from build123d import *

# Parameters (mm, degrees)
CROQUIS1_R              = 27.5
CROQUIS1_R_2            = 19.05
SALIENTE_EXTRUIR1_DEPTH = 3
CORTAR_EXTRUIR1_DEPTH   = 3


with BuildPart() as part:
    # Croquis1 → Saliente-Extruir1 (new body)
    with BuildSketch(Plane(origin=(0, 0, 0), x_dir=(1, 0, 0), z_dir=(0, 1, 0))):
        Circle(CROQUIS1_R)
        Circle(CROQUIS1_R_2, mode=Mode.SUBTRACT)
    extrude(amount=SALIENTE_EXTRUIR1_DEPTH)

    # Croquis2 → Cortar-Extruir1 (cut)
    with BuildSketch(Plane(origin=(0, 3, 0), x_dir=(1, 0, 0), z_dir=(0, 1, 0))):
        Polygon((-1.170833669, -27.475064122), (-3.980970396, -18.629395447), (-1.170833669, -17.73665701), (2.334832716, -28.771694214), (-0.475304011, -29.664432651), align=None)
    extrude(amount=-CORTAR_EXTRUIR1_DEPTH, mode=Mode.SUBTRACT)


solid = part.part
Model file for the job. Use its own axes, mm. Coordinates: 2 decimals unless noted, no trailing zeros. Loops run counter-clockwise (first coordinate to the right, second up) from the corner with the lowest first, then second, coordinate; pieces in that order, holes last. Notation, with made-up numbers: (-3, -32.75) -> (52, -32.75) arc R22 cw to (52, 1.25) -> close; hole circle Ø5 at (-16.5, 48). An arc over 180 degrees is marked (long way). Use one line per item in the form item = value. Start each with the question number.
(1) Flat gauge pin, fed straight in: pin 1 (8 mm diameter, centred on x = 14, z = -6.5, fed in from +Y). Where does the tip first touch, or does it go through?
(2) Cut at D-D on z = -23. Give the cut face in (x, y).
(3) Cut at C-C on y = 2.1. Give the cut face in (x, z).
(4) Probe probe 1 along X at (y, z) = (0.7, 0.5); probe 2 along X at (y, z) = (0.6, 11.5); probe 3 along Z at (x, y) = (-9, 1.6). List the from-to ranges inside material, lowest first. Write a range as from..to.
(5) Pull direction Z, two halves, no side cores. Call faces 1 (the flat face through (-19, 0, 6)), 2 (the flat face through (0.56, 1.52, 23.18)), 3 (the flat face through (-2.556, 1.521, 23.114)): pulls with the +Z half, pulls with the -Z half, needs draft (parallel to the pull), parting line crosses it, or undercut.
(6) Cut at A-A on z = -9. Give the cut face in (x, y), and give its area (3 significant figures).
(7) Cut at B-B on x = 0. Give the cut face in (y, z), and give its area (3 significant figures).
Values:
q1.pin_1 = 3
q2.outline = (-15.07, 0) -> (15.07, 0) -> (15.07, 3) -> (-15.07, 3) -> close
q3.outline = (-3.98, 18.63) -> (-1.17, 27.48) arc R27.5 ccw (long way) to (1.91, 27.43) -> (-0.76, 19.03) arc R19.05 cw (long way) to start
q4.probe_1 = -27.5..-19.04, 19.04..27.5
q4.probe_2 = -24.98..-15.19, 15.19..24.98
q4.probe_3 = -25.99..-16.79, 16.79..25.99
q5.face_1 = needs draft
q5.face_2 = pulls with the +Z half
q5.face_3 = undercut
q6.outline = (-25.99, 0) -> (-16.79, 0) -> (-16.79, 3) -> (-25.99, 3) -> close; (16.79, 0) -> (25.99, 0) -> (25.99, 3) -> (16.79, 3) -> close
q6.area = 55.2 mm2
q7.outline = (0, -27.5) -> (3, -27.5) -> (3, -19.05) -> (0, -19.05) -> close; (0, 19.05) -> (3, 19.05) -> (3, 21.42) -> (0, 21.42) -> close
q7.area = 32.5 mm2
